Could you check a few things on this model? Use its own coordinates, in mm. A direction names the side the tool comes from. Round coordinates to 2 decimals unless told otherwise and drop trailing zeros. Write each loop counter-clockwise with the first axis right and the second up, starting at its lowest first coordinate (ties: lowest second). Pieces come first, ordered by that corner, then holes. Notation, with made-up numbers: (56.25, 45.25) -> (66.25, 45.25) arc R11 cw to (66.25, 56.25) -> close; hole circle Ø5 at (89.5, 37). An arc over 180 degrees is marked (long way). Return JSON: item names as keys, results as strings.
Autodesk Inventor part; units mm, degrees
ref_plane "YZ Plane" through (0, 0, 0) normal (1, 0, 0) x (0, 1, 0)
ref_plane "XZ Plane" through (0, 0, 0) normal (0, 1, 0) x (-1, 0, 0)
ref_plane "XY Plane" through (0, 0, 0) normal (0, 0, 1) x (1, 0, 0)
sketch "Sketch1" plane through (0, 0, 0) normal (0, 0, 1) x (1, 0, 0)
  circle A0 centre (0, 0) radius 8
  dimension "d0" = 16
extrude "Extrusion1" add sketch "Sketch1" along normal blind 5.5
sketch "Sketch2" plane through (0, 0, 5.5) normal (0, 0, 1) x (1, 0, 0)
  circle A0 centre (0, 0) radius 7.5
  dimension "d3" = 15
extrude "Extrusion2" add sketch "Sketch2" along normal blind 20.1
sketch "Sketch3" plane through (0, 0, 0) normal (0, 0, -1) x (-1, 0, 0)
  circle A0 centre (0, 0) radius 1.5
  dimension "d6" = 3
extrude "Extrusion3" add sketch "Sketch3" along normal blind 6
sketch "Sketch4" plane through (0, 0, 25.6) normal (0, 0, 1) x (1, 0, 0)
  point P0 (0, 0)
  point P1 (0.0077, 0.354)
hole "Hole1" at (0.0077, 0.354, 25.6) direction (0, 0, -1) diameter 11.4587 depth 24
properties part number "shaft"
1) Will these pins go through, and if not, where does the flat tip stop? pin 1 Ø6 at (x, z) = (1.5, 13) entering from +Y; pin 2 Ø4 at (x, z) = (6, 21.5) entering from +Y; pin 3 Ø4 at (x, z) = (0, 18.5) entering from -Y.
Return value:
{"pin 1": "y = 7.5", "pin 2": "y = 6.34", "pin 3": "y = -7.5"}
2) I want a section at B-B, the plane z = 16.5. Please give me the cut outline in (x, y), and give its area (3 significant figures).
Return value:
{"outline": "circle Ø15 at (0, 0); hole circle Ø11.46 at (0.01, 0.35)", "area": "73.6 mm²"}
3) If I drill on probe 1 along Z at (x, y) = (-2.25, 3.5); probe 2 along Z at (x, y) = (-0.75, 1.25); probe 3 along Y at (x, z) = (0.5, 19), over which ranges is the centre line in solid material (lowest first)? Write a range as [from, to].
Return value:
{"probe 1": "[0, 1.6]", "probe 2": "[-6, 1.6]", "probe 3": "[-7.48, -5.35], [6.06, 7.48]"}
4) Thinking about a two-plate mould opening in Y: for faces 1 (the face through (0, 0, -6)), 2 (the face through (-1.71, -5.11, 13.43)), 3 (the face through (-7.493, -0.33, 15.409)), which applies, pulls with the +Y half, pulls with the -Y half, needs draft (parallel to the pull), parting line crosses it, or undercut?
Return value:
{"face 1": "needs draft", "face 2": "undercut", "face 3": "parting line crosses it"}
5) For faces 4 (the face through (0, 0, 1.6)), 5 (the face through (1.5, -0.07, -2.96)), 6 (the face through (-1.73, 7.81, 2.71)), which set-ups out of +Z, -Z, +X, -X, +Y, -Y let a thin tool reach every point of the face, with its end or its side?
Return value:
{"face 4": "+Z", "face 5": "-Z", "face 6": "+Z, -Z"}
6) I want a section at C-C, the plane y = 0. Please give me the cut outline in (x, z), and give its area (3 significant figures).
Return value:
{"outline": "(-8, 0) -> (-1.5, 0) -> (-1.5, -6) -> (1.5, -6) -> (1.5, 0) -> (8, 0) -> (8, 5.5) -> (7.5, 5.5) -> (7.5, 25.6) -> (5.73, 25.6) -> (5.73, 1.6) -> (-5.71, 1.6) -> (-5.71, 25.6) -> (-7.5, 25.6) -> (-7.5, 5.5) -> (-8, 5.5) -> close", "area": "133 mm²"}
7) I want a section at A-A, the plane y = -6.5. Please give me the cut outline in (x, z).
Return value:
{"outline": "(-4.66, 0) -> (4.66, 0) -> (4.66, 5.5) -> (3.74, 5.5) -> (3.74, 25.6) -> (-3.74, 25.6) -> (-3.74, 5.5) -> (-4.66, 5.5) -> close"}
8) I want a section at D-D, the plane y = 2.25. Please give me the cut outline in (x, z).
Return value:
{"outline": "(-7.68, 0) -> (7.68, 0) -> (7.68, 5.5) -> (7.15, 5.5) -> (7.15, 25.6) -> (5.41, 25.6) -> (5.41, 1.6) -> (-5.4, 1.6) -> (-5.4, 25.6) -> (-7.15, 25.6) -> (-7.15, 5.5) -> (-7.68, 5.5) -> close"}
